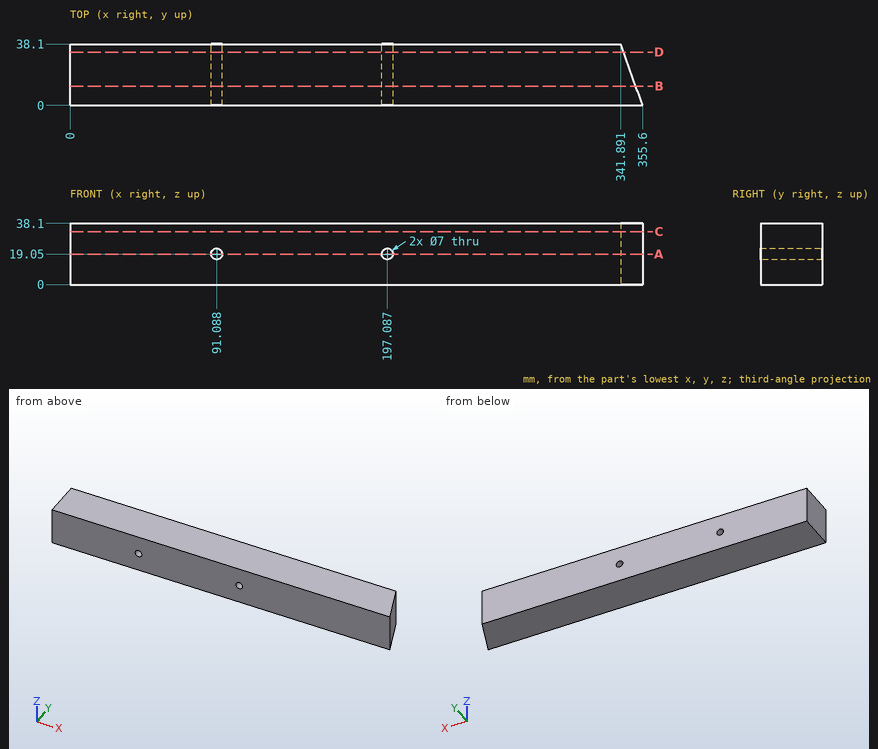
Answer from the drawing. Dimensions are ordinates in mm from the lowest x, y and z of the part. Round coordinates to 2 decimals unless told otherwise and drop trailing zeros. Write each loop counter-clockwise with the first axis right and the second up, starting at its lowest first coordinate (ties: lowest second). Pieces come first, ordered by that corner, then holes.
1. The part is cut by section C-C, the plane z = 33. Determine the outline of the cut face in (x, y).
2. Given pin 1 Ø4 at (x, z) = (91.09, 19.05) entering from +Y; pin 2 Ø8 at (y, z) = (30.5, 11.5) entering from +X (1 decimal); pin 3 Ø1.5 at (y, z) = (31, 20) entering from +X (1 decimal), each flat-ended and moving along its own axis, determine where each tip first touches the part or whether it passes through.
3. The part is cut by section D-D, the plane y = 33. State how many separate pieces and enclosed holes the cut face has, then the cut area to 3 significant figures.
4. The part is cut by section A-A, the plane z = 19.05. Determine the outline of the cut face in (x, y).
5. The part is cut by section B-B, the plane y = 12. Determine the outline of the cut face in (x, z), then the cut area to 3 significant figures.
6. Straight lines are drawn through the part: L1, parallel to X at y = 22, z = 19 (1 decimal); L2, parallel to X at y = 20, z = 19; L3, parallel to Z at x = 94, y = 28 (1 decimal). For each, find the intervals that lie inside material, in ascending order.
Values:
1. outline: (0, 0) - (355.6, 0) - (341.89, 38.1) - (0, 38.1) - close
2. pin 1: passes through
2. pin 2: stops at x = 346.1
2. pin 3: stops at x = 344.7
3. separate pieces: 1
3. enclosed holes: 2
3. area: 13,000 mm2
4. outline: (0, 0) - (87.59, 0) - (87.59, 38.1) - (0, 38.1) - close; (94.59, 0) - (193.59, 0) - (193.59, 38.1) - (94.59, 38.1) - close; (200.59, 0) - (355.6, 0) - (341.89, 38.1) - (200.59, 38.1) - close
5. outline: (0, 0) - (351.28, 0) - (351.28, 38.1) - (0, 38.1) - close; hole circle Ø7 at (91.09, 19.05); hole circle Ø7 at (197.09, 19.05)
5. area: 13,300 mm2
6. L1: x = 0 to 87.6, 94.6 to 193.6, 200.6 to 347.7
6. L2: x = 0 to 87.59, 94.59 to 193.59, 200.59 to 348.4
6. L3: z = 0 to 17.1, 21 to 38.1
